Input: part model. Units: mm. Frame: model coordinates. Face numbers are marked on the shaded views. A direction names the side the tool comes from. Give positions to 0.01 mm unless a question says otherwise; leave off trailing zeros. Write each loop counter-clockwise with the first axis right and the second up, starting at its lowest first coordinate (ties: lowest second). Pieces come first, ordered by that corner, then holes. Notation, with made-up numbers: (46, 48) - (60, 48) arc R18 ccw to (60, 61) - close; hole circle Ø8 at (4, -33.75). An arc over 180 degrees is marked (long way). Use a Markdown table: item, result. Add a question column.
1. Pin query (flat end, axial travel): pin 1 (6 mm diameter, centred on x = 4, z = -24.5, fed in from +Y); pin 2 (6.5 mm diameter, centred on x = 5, z = -45.005, fed in from -Y); pin 3 (2 mm diameter, centred on x = 10.5, z = 4.5, fed in from +Y). Return the tip coordinate at first contact, or that it passes through.
2. Set-up query: the marked faces 1, 2 and 3. Return all of +Z, -Z, +X, -X, +Y, -Y with unobstructed straight access to the full face (end or side cutting, diameter ignored); none if empty.
3. Material intervals for probe 1 along Y at (x, z) = (13.25, 2); probe 2 along Z at (x, y) = (15, 29.1) (3 decimals); probe 3 along Y at (x, z) = (1, -15), sorted ascending.
4. Mould query, pull axis Z, two halves, no side actions, for the marked faces 4, 5 and 6. Classes: released by +Z, released by -Z, zero draft, split by the parting line, or undercut.
5. Section query C-C, the plane y = 33. Return loops of the section in (x, z).
6. Section query A-A, the plane y = 3.5. Return loops of the section in (x, z).
7. Section query B-B, the plane z = -31. Return loops of the section in (x, y).
```python
from build123d import *

# Parameters (mm, degrees)
SKETCH1_W                = 20
SKETCH1_H                = 40
BOSS_EXTRUDE1_DEPTH      = 36
SKETCH2_W                = 7
SKETCH2_H                = 3
BOSS_EXTRUDE2_DEPTH      = 5
SKETCH3_R                = 2.5
BOSS_EXTRUDE3_DEPTH      = 8.5
BOSS_EXTRUDE4_DEPTH      = 7
BOSS_EXTRUDE4_DEPTH_BACK = 47
SKETCH4_W                = 20
SKETCH4_H                = 2.5
SKETCH5_R                = 2
CUT_EXTRUDE1_DEPTH       = 7
BOSS_EXTRUDE5_DEPTH      = 2
SKETCH7_R                = 6.289454611
BOSS_EXTRUDE6_DEPTH      = 1
FILLET1_R                = 1
FILLET2_R                = 1
SKETCH8_R                = 1.25
CUT_EXTRUDE2_DEPTH       = 5


with BuildPart() as part:
    # Sketch1 → Boss-Extrude1 (new body)
    with BuildSketch(Plane(origin=(0, 0, 0), x_dir=(1, 0, 0), z_dir=(0, 1, 0))):
        with Locations((10, 20)):
            Rectangle(SKETCH1_W, SKETCH1_H)
    extrude(amount=BOSS_EXTRUDE1_DEPTH)

    # Sketch2 → Boss-Extrude2 (add)
    with BuildSketch(Plane.XY):
        with Locations((10, 4)):
            Rectangle(SKETCH2_W, SKETCH2_H)
    extrude(amount=BOSS_EXTRUDE2_DEPTH)

    # Sketch3 → Boss-Extrude3 (add)
    with BuildSketch(Plane(origin=(0, 36, 0), x_dir=(1, 0, 0), z_dir=(0, 1, 0))):
        with Locations(Location((10, 10, 0), (0, 0, 90))):
            Circle(SKETCH3_R)
    extrude(amount=BOSS_EXTRUDE3_DEPTH)

    # Sketch4 → Boss-Extrude4 (add, two sides: drawn at the far end of the back side and taken through both)
    with BuildSketch(Plane.XY.offset(-BOSS_EXTRUDE4_DEPTH_BACK)):
        with Locations((10, 29.25)):
            Rectangle(SKETCH4_W, SKETCH4_H)
    extrude(amount=BOSS_EXTRUDE4_DEPTH + BOSS_EXTRUDE4_DEPTH_BACK)

    # Sketch5 → Cut-Extrude1 (cut)
    with BuildSketch(Plane(origin=(0, 30.5, 0), x_dir=(1, 0, 0), z_dir=(0, 1, 0))):
        with Locations((15, 45.005)):
            Circle(SKETCH5_R)
        with Locations((5, 45.005)):
            Circle(SKETCH5_R)
        with Locations((15, -5.005)):
            Circle(SKETCH5_R)
        with Locations((5, -5.005)):
            Circle(SKETCH5_R)
    extrude(amount=-CUT_EXTRUDE1_DEPTH, mode=Mode.SUBTRACT)

    # Sketch6 → Boss-Extrude5 (add)
    with BuildSketch(Plane(origin=(0, 36, 0), x_dir=(1, 0, 0), z_dir=(0, 1, 0))):
        with BuildLine():
            Line((20, 32.5), (13.5, 32.5))
            ThreePointArc((13.5, 32.5), (10, 36), (6.5, 32.5))
            Line((6.5, 32.5), (0, 32.5))
            Line((0, 32.5), (0, 10))
            ThreePointArc((0, 10), (10, 0), (20, 10))
            Line((20, 10), (20, 32.5))
        make_face()
    extrude(amount=BOSS_EXTRUDE5_DEPTH)

    # Sketch7 → Boss-Extrude6 (add)
    with BuildSketch(Plane(origin=(0, 38, 0), x_dir=(1, 0, 0), z_dir=(0, 1, 0))):
        with Locations(Location((10, 10, 0), (0, 0, 270))):
            Circle(SKETCH7_R)
    extrude(amount=BOSS_EXTRUDE6_DEPTH)

    # Fillet1
    fillet1_edges = [part.edges().sort_by_distance(p)[0] for p in [
        (10, 39, -16.289454611),
    ]]
    fillet(fillet1_edges, radius=FILLET1_R - 0.0001)  # a hair under: the kernel refuses the full size

    # Fillet2
    fillet2_edges = [part.edges().sort_by_distance(p)[0] for p in [
        (10, 38, -36),
    ]]
    fillet(fillet2_edges, radius=FILLET2_R)

    # Sketch8 → Cut-Extrude2 (cut)
    with BuildSketch(Plane(origin=(0, 44.5, 0), x_dir=(1, 0, 0), z_dir=(0, 1, 0))):
        with Locations(Location((10, 10, 0), (0, 0, 270))):
            Circle(SKETCH8_R)
    extrude(amount=-CUT_EXTRUDE2_DEPTH, mode=Mode.SUBTRACT)


solid = part.part
```
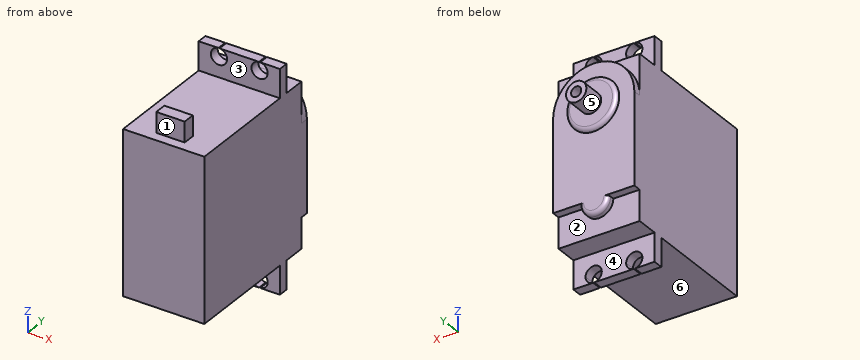
Result sheet:
| question | item | result |
|---|---|---|
| 1 | pin 1 | stops at y = 38 |
| 1 | pin 2 | stops at y = 28 |
| 1 | pin 3 | stops at y = 30.5 |
| 2 | face 1 | +Z, +X, -X, -Y |
| 2 | face 2 | -Z, +Y |
| 2 | face 3 | +Z, +X, -X |
| 3 | probe 1 | y = 2.5 to 5.5, 28 to 30.5 |
| 3 | probe 2 | z = -43.005 to 3.005 |
| 3 | probe 3 | y = 0 to 38 |
| 4 | face 4 | zero draft |
| 4 | face 5 | split by the parting line |
| 4 | face 6 | released by -Z |
| 5 | outline | (0, -40) - (20, -40) - (20, 0) - (0, 0) - close |
| 6 | outline | (0, -40) - (20, -40) - (20, 0) - (13.5, 0) - (13.5, 5) - (6.5, 5) - (6.5, 0) - (0, 0) - close |
| 7 | outline | (0, 0) - (20, 0) - (20, 38) - (0, 38) - close |
